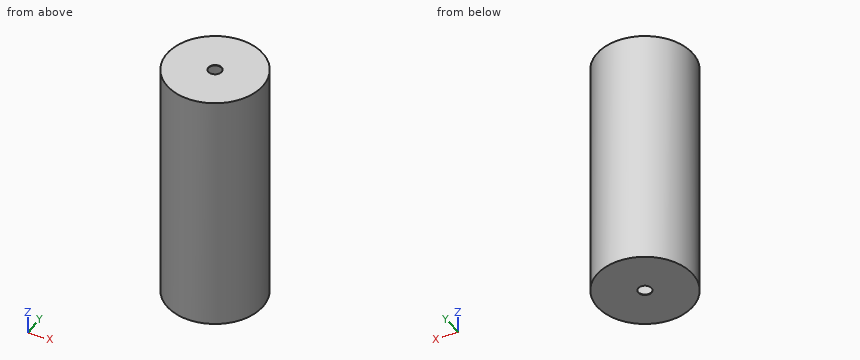
```python
from build123d import *

# Parameters (mm, degrees)
SKETCH3_R          = 1.1
CUT_EXTRUDE1_DEPTH = 53


# Read off the part's stored shape, not the designer's step: Extrude-Thin1
with BuildPart() as part:
    # Extrude-Thin1 outline → Extrude-Thin1 (revolve)
    with BuildSketch(Plane.XZ):
        Polygon((7.9, 40.4), (0, 40.4), (0, 40.3), (7.8, 40.3), (7.8, 0.1), (0, 0.1), (0, 0), (7.9, 0), align=None)
    revolve(axis=Axis((0, 0, 0), (0, 0, 1)))

    # Sketch3 → Cut-Extrude1 (cut)
    with BuildSketch(Plane(origin=(0, 0, 0), x_dir=(-1, 0, 0), z_dir=(0, 0, -1))):
        Circle(SKETCH3_R)
    extrude(amount=-CUT_EXTRUDE1_DEPTH, mode=Mode.SUBTRACT)


solid = part.part
```
For this review, take the finished solid that the model builds, in its own axes (mm). Round coordinates to 2 decimals unless told otherwise and drop trailing zeros. Write each loop counter-clockwise with the first axis right and the second up, starting at its lowest first coordinate (ties: lowest second). Pieces come first, ordered by that corner, then holes.
1) Take a section at C-C on y = -2. Give the boundary of the cut face in (x, z).
Answer below:
outline: (-7.64, 0) - (7.64, 0) - (7.64, 40.4) - (-7.64, 40.4) - close; hole (-7.54, 0.1) - (7.54, 0.1) - (7.54, 40.3) - (-7.54, 40.3) - close
2) Insertion check: pin 1 Ø4.5 at (x, y) = (-2.5, 0) entering from -Z; pin 2 Ø4 at (x, z) = (2.5, 32.5) entering from -Y; pin 3 Ø5 at (y, z) = (5.5, 11) entering from +X; pin 4 Ø1.5 at (y, z) = (4, 22.5) entering from +X. Each pin has a flat end and moves straight along its axis. Give the tip position at first contact, or say it passes through.
Answer below:
pin 1: stops at z = 0
pin 2: stops at y = -7.88
pin 3: stops at x = 7.31
pin 4: stops at x = 7.2
3) Take a section at D-D on x = -6.5. Give the boundary of the cut face in (y, z), then the cut area to 3 significant figures.
Answer below:
outline: (-4.49, 0) - (4.49, 0) - (4.49, 40.4) - (-4.49, 40.4) - close; hole (-4.31, 0.1) - (4.31, 0.1) - (4.31, 40.3) - (-4.31, 40.3) - close
area: 16.1 mm2
4) For line 1 along Y through (x, z) = (0, 0.05), list the stretches that pass through material, from the lowest coordinate up.
Answer below:
line 1: y = -7.9 to -1.1, 1.1 to 7.9
5) Take a section at A-A on y = 0. Give the boundary of the cut face in (x, z), then the cut area to 3 significant figures.
Answer below:
outline: (-7.9, 0) - (-1.1, 0) - (-1.1, 0.1) - (-7.8, 0.1) - (-7.8, 40.3) - (-1.1, 40.3) - (-1.1, 40.4) - (-7.9, 40.4) - close; (1.1, 0) - (7.9, 0) - (7.9, 40.4) - (1.1, 40.4) - (1.1, 40.3) - (7.8, 40.3) - (7.8, 0.1) - (1.1, 0.1) - close
area: 10.8 mm2
